from build123d import *

# Parameters (mm, degrees)
F1_DEPTH = 1219.2


with BuildPart() as f1:
    # F0 (on Right) → F1 (new body)
    with BuildSketch(Plane.YZ):
        Polygon((0, -32.372466), (0, 0), (-32.372466, 0), (-32.372466, -4.772527), (-4.772527, -4.772527), (-4.772527, -32.372466), align=None)
        Polygon((32.372466, 0), (0, 0), (0, -32.372466), (4.772527, -32.372466), (4.772527, -4.772527), (32.372466, -4.772527), align=None)
    extrude(amount=F1_DEPTH)


solid = f1.part
Could you check a few things on this model? Use its own coordinates, in mm. A direction names the side the tool comes from. Coordinates: 2 decimals unless noted, no trailing zeros. Order: outer loops, then holes, each group sorted by start corner. A loop starts at its lowest first (then second) coordinate and runs counter-clockwise, first axis right, second up. Notation, with made-up numbers: (84.5, -21) -> (91.5, -21) arc R24 cw to (91.5, -2) -> close; hole circle Ø5 at (86.5, 88.5). An arc over 180 degrees is marked (long way). One line per question, with ' | ' between items.
Q1. Imagine slicing it at B-B on y = 21. Please give me the cut outline in (x, z).
Return value:
outline: (0, -4.77) -> (1219.2, -4.77) -> (1219.2, 0) -> (0, 0) -> close
Q2. On a 3-axis mill with a long thin cutter (end or side, diameter ignored), from which of +Z, -Z, +X, -X, +Y, -Y can I reach the whole of each face in a straight line? I mean faces 1 (the face through (601, 18, -4.773)), 2 (the face through (601, -19, -4.773)), 3 (the face through (601, 0, 0)). Say none if no direction works.
Return value:
face 1: -Z, +X, -X, +Y | face 2: -Z, +X, -X, -Y | face 3: +Z, +X, -X, +Y, -Y
Q3. I'm going to push flat-ended pins straight in: P1, Ø14, axis at x = 552, y = -16, coming from the -Z side; P2, Ø2, axis at x = 662, z = -28.5, coming from the +Y side. Where does each tip first touch, or does it pass through?
Return value:
P1: z = -4.77 | P2: y = 4.77
Q4. If I drill on L1, parallel to Z at x = 140.5, y = -16; L2, parallel to Y at x = 714.5, z = -16, over which ranges is the centre line in solid material (lowest first)?
Return value:
L1: -4.77 to 0 | L2: -4.77 to 4.77
Q5. Imagine slicing it at C-C on z = -14. Please give me the cut outline in (x, y), and give its area (3 significant figures).
Return value:
outline: (0, -4.77) -> (1219.2, -4.77) -> (1219.2, 4.77) -> (0, 4.77) -> close | area: 11,600 mm²
Q6. Imagine slicing it at A-A on x = 1073.5. Please give me the cut outline in (y, z).
Return value:
outline: (-32.37, -4.77) -> (-4.77, -4.77) -> (-4.77, -32.37) -> (4.77, -32.37) -> (4.77, -4.77) -> (32.37, -4.77) -> (32.37, 0) -> (-32.37, 0) -> close
